Autodesk Inventor part; units mm, degrees
ref_plane "Work Plane1" through (30.1625, 0, 0) normal (0, 0, -1) x (1, 0, 0)
ref_plane "YZ Plane" through (0, 0, 0) normal (1, 0, 0) x (0, 1, 0)
ref_plane "XZ Plane" through (0, 0, 0) normal (0, 1, 0) x (-1, 0, 0)
sketch "Sketch1" plane through (0, 0, 0) normal (0, 0, 1) x (1, 0, 0)
  line L0 (-6, 0) -> (60, 0)
  line L1 (60, 0) -> (60, 5)
  line L2 (60, 5) -> (22, 5)
  line L3 (22, 5) -> (21.0797, 4.54)
  line L4 (21.0797, 4.54) -> (0, 4.54)
  line L5 (0, 4.54) -> (0, 8)
  line L6 (-19.2, 0) -> (73.2, 0)
  line L7 (0, -1.6) -> (0, 9.6)
  line L8 (-6, 0) -> (-6, 7.4751)
  line L9 (0, 8) -> (-6, 7.4751)
  line L10 (22, 5) -> (0, 5) construction
  dimension "d0" = 60
  dimension "d1" = 38
  dimension "d2" = 0.9203
  dimension "d3" = 6
  dimension "d4" = 10
  dimension "d5" = 9.08
  dimension "d9" = 16
  dimension "d10" = 5
revolve "Body" add sketch "Sketch1" angle 360 about axis through (-6, 0, 0) along (1, 0, 0)
sketch "Sketch2" plane through (-6, 0, 0) normal (-1, 0, 0) x (0, 0, 1)
  circle A0 centre (0, 0) radius 8
  line L0 (0, 0) -> (0, 7.4751)
  line L1 (-8, 1.25) -> (8, 1.25)
  line L2 (8, 1.25) -> (8, -1.25)
  line L3 (8, -1.25) -> (-8, -1.25)
  line L4 (-8, -1.25) -> (-8, 1.25)
  line L5 (-8, 0) -> (8, 0) construction
  line L6 (0, 1.25) -> (0, -1.25) construction
  dimension "d11" = 2.5
  dimension "d12" = 16
fillet "Fillet1" radius 0.4 1 edges at (-6, -7.4751, 0)
extrude "Slot" cut sketch "Sketch2" against normal blind 2.4 contours A0 L3 L1 | L2 L3 A0 | A0 L1 L2 | A0 L4 L1 | L3 L4 A0
thread "Thread"
chamfer "Chamfer1" distance 0.9202 distance2 0.9203 1 edges at (60, -5, 0) measured on face at (60, -0.01, -0.88)
ref_plane "Work Plane1" through (30.1625, 0, 0) normal (0, 0, -1) x (1, 0, 0)
equation "\"d11\" = SBR"
equation "\"d12\" = KOD"
equation "\"d19\" = STI"
equation "\"d14\" = RR"
equation "\"d15\" = GEL"
equation "\"d17\" = -0.5 * SPD + 0.5 * GD"
equation "\"d0\" = NLG"
equation "\"d1\" = GEL"
equation "\"d3\" = KOH"
equation "\"d4\" = GD"
equation "\"d5\" = BDM"
equation "\"d9\" = KOD"
equation "\"d10\" = KEWI"
equation "\"GD\" = NND"
equation "\"NLG\" = 60"
equation "\"GEL\" = 38"
equation "\"KOD\" = 16"
equation "\"KOH\" = 6"
equation "\"GAL\" = 0.61345 * PTC"
equation "\"SPD\" = NND - 1.2269 * PTC"
equation "\"BDM\" = 9.08"
equation "\"GUL\" = 0.61345 * PTC"
equation "\"RR\" = 0.4"
equation "\"SBR\" = 2.5"
equation "\"STI\" = 2.4"
equation "\"KEWI\" = 5deg"
equation "\"PTC\" = 1.5"
equation "\"TOA\" = 30deg"
equation "\"GD1\" = THREADDIA - 1.2269 * PTC"
properties part number "ISO 1207 - M10 x 60" material "Stainless Steel, 440C"
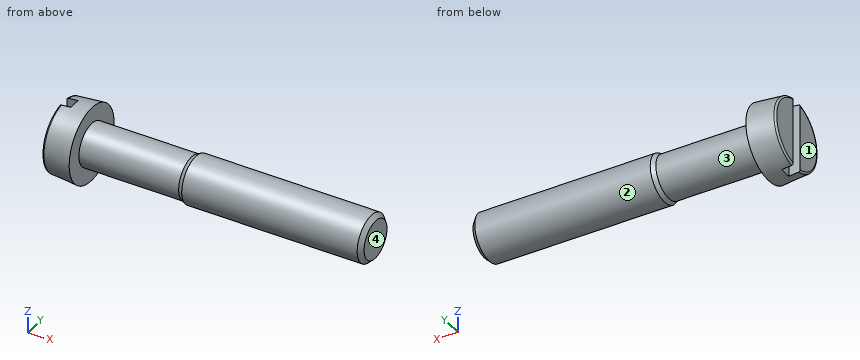
For this review, take the finished solid that the model builds, in its own axes (mm). Face numbers are marked on the shaded views. Coordinates: 2 decimals unless noted, no trailing zeros. Loops run counter-clockwise (first coordinate to the right, second up) from the corner with the lowest first, then second, coordinate; pieces in that order, holes last. Notation, with made-up numbers: (-11, 9) -> (-2, 9) arc R24 cw to (-2, 20) -> close; hole circle Ø7 at (39.25, 78). An arc over 180 degrees is marked (long way). Return JSON: item names as keys, results as strings. Group by question number.
(1) Consider section D-D, the plane x = 7. Give the boundary of the cut face in (y, z), plus the area to 3 significant figures.
(2) Mouldability with a two-part tool opening along X and no side actions: class the marked faces 1, 2, 3 and 4 as pulls with the +X half, pulls with the -X half, needs draft (parallel to the pull), parting line crosses it, or undercut.
(3) Consider section C-C, the plane x = 56. Give the boundary of the cut face in (y, z).
(4) For pin 1 Ø2 at (x, z) = (16, -5) entering from -Y; pin 2 Ø6 at (x, y) = (51.5, 6.5) entering from -Z; pin 3 Ø6 at (x, z) = (49, -0.5) entering from +Y; pin 4 Ø2 at (y, z) = (-0.5, -3.5) entering from -X, all flat-tipped, find the tip position at first contact; note any pin that passes through.
(5) Consider section B-B, the plane z = 0. Give the boundary of the cut face in (x, y), plus the area to 3 significant figures.
(6) To check wall thickness, follow L1, parallel to X at y = 1, z = 6.75; L2, parallel to X at y = 0.75, z = -2.75; L3, parallel to Y at x = 9, z = -1. State the ranges of each line that lie inside material, in increasing order.
(7) Consider section A-A, the plane y = 0. Give the boundary of the cut face in (x, z).
Results below:
{
 "1": {"outline": "circle Ø9.08 at (0, 0)", "area": "64.8 mm2"},
 "2": {"face 1": "pulls with the -X half", "face 2": "needs draft", "face 3": "undercut", "face 4": "pulls with the +X half"},
 "3": {"outline": "circle Ø10 at (0, 0)"},
 "4": {"pin 1": "stops at y = -2.15", "pin 2": "stops at z = -3.57", "pin 3": "stops at y = 5", "pin 4": "stops at x = -6"},
 "5": {"outline": "(-6, -7.11) arc R0.4 ccw to (-5.63, -7.51) -> (0, -8) -> (0, -4.54) -> (21.08, -4.54) -> (22, -5) -> (59.08, -5) -> (60, -4.08) -> (60, 4.08) -> (59.08, 5) -> (22, 5) -> (21.08, 4.54) -> (0, 4.54) -> (0, 8) -> (-5.63, 7.51) arc R0.4 ccw to (-6, 7.11) -> (-6, 1.25) -> (-3.6, 1.25) -> (-3.6, -1.25) -> (-6, -1.25) -> close", "area": "666 mm2"},
 "6": {"L1": "x = -3.6 to 0", "L2": "x = -3.6 to 60", "L3": "y = -4.43 to 4.43"},
 "7": {"outline": "(-3.6, -7.69) -> (0, -8) -> (0, -4.54) -> (21.08, -4.54) -> (22, -5) -> (59.08, -5) -> (60, -4.08) -> (60, 4.08) -> (59.08, 5) -> (22, 5) -> (21.08, 4.54) -> (0, 4.54) -> (0, 8) -> (-3.6, 7.69) -> close"}
}
